from build123d import *

# Parameters (mm, degrees)
SKETCH_1_R          = 2
SKETCH_1_W          = 26
SKETCH_1_H          = 26
EXTRUDE_1_DEPTH     = 5
EXTRUDE_2_DEPTH     = 24
EXTRUDE_3_DEPTH     = 32
CUT_EXTRUDE_1_REACH = 71.979
SKETCH_3_R          = 6.35
CUT_EXTRUDE_2_REACH = 67.49
SKETCH_4_R          = 6.35
FILLET_2_R          = 3


with BuildPart() as part:
    # Sketch 1 → Extrude 1 (new body)
    with BuildSketch(Plane(origin=(0, 0, 0), x_dir=(1, 0, 0), z_dir=(0, 1, 0))):
        with BuildLine():
            Line((3, 0), (39, 0))
            ThreePointArc((39, 0), (41.121320344, 0.878679656), (42, 3))
            Line((42, 3), (42, 39))
            ThreePointArc((42, 39), (41.121320344, 41.121320344), (39, 42))
            Line((39, 42), (3, 42))
            ThreePointArc((3, 42), (0.878679656, 41.121320344), (0, 39))
            Line((0, 39), (0, 3))
            ThreePointArc((0, 3), (0.878679656, 0.878679656), (3, 0))
        make_face()
        with Locations(Location((5, 37, 0), (0, 0, 270))):
            Circle(SKETCH_1_R, mode=Mode.SUBTRACT)
        with Locations(Location((39, 37, 0), (0, 0, 270))):
            Circle(SKETCH_1_R, mode=Mode.SUBTRACT)
        with Locations(Location((5, 3, 0), (0, 0, 270))):
            Circle(SKETCH_1_R, mode=Mode.SUBTRACT)
        with Locations((21, 21)):
            Rectangle(SKETCH_1_W, SKETCH_1_H, mode=Mode.SUBTRACT)
    extrude(amount=EXTRUDE_1_DEPTH)

    # Sketch 2 → Extrude 2 (add)
    with BuildSketch(Plane(origin=(0, 5, 0), x_dir=(1, 0, 0), z_dir=(0, 1, 0))):
        Polygon((35.65, 34), (35.65, 42), (11.65, 42), (11.65, 34), (34, 34), align=None)
    extrude(amount=EXTRUDE_2_DEPTH)

    # Sketch 2_3 → Extrude 3 (add)
    with BuildSketch(Plane(origin=(0, 5, 0), x_dir=(1, 0, 0), z_dir=(0, 1, 0))):
        Polygon((8, 30.35), (0, 30.35), (0, 6.35), (8, 6.35), (8, 8), align=None)
    extrude(amount=EXTRUDE_3_DEPTH)

    # Sketch 3 → Cut-Extrude 1 (cut, up to next)
    with BuildSketch(Plane(origin=(0, 0, -42), x_dir=(-1, 0, 0), z_dir=(0, 0, -1)), mode=Mode.PRIVATE) as cut_extrude_1_sk1:
        with Locations((-25.65, 20)):
            Circle(SKETCH_3_R)
    cut_extrude_1_tool1 = extrude(cut_extrude_1_sk1.sketch, amount=-CUT_EXTRUDE_1_REACH, mode=Mode.PRIVATE) & part.part
    # Sketch 3 → Cut-Extrude 1 (cut, up to next)
    with BuildSketch(Plane(origin=(0, 0, -42), x_dir=(-1, 0, 0), z_dir=(0, 0, -1)), mode=Mode.PRIVATE) as cut_extrude_1_sk2:
        with BuildLine():
            Line((-30.008898944, 29), (-35.65, 29))
            Line((-35.65, 29), (-35.65, 20))
            ThreePointArc((-35.65, 20), (-34.123163206, 25.310885546), (-30.008898944, 29))
        make_face()
    cut_extrude_1_tool2 = extrude(cut_extrude_1_sk2.sketch, amount=-CUT_EXTRUDE_1_REACH, mode=Mode.PRIVATE) & part.part
    add(cut_extrude_1_tool1.solids().sort_by_distance((25.65, 20, -42))[0], mode=Mode.SUBTRACT)
    add(cut_extrude_1_tool2.solids().sort_by_distance((34.089564, 26.895646, -42))[0], mode=Mode.SUBTRACT)

    # Sketch 4 → Cut-Extrude 2 (cut, up to next)
    with BuildSketch(Plane(origin=(8, 0, 0), x_dir=(0, 0, -1), z_dir=(1, 0, 0)), mode=Mode.PRIVATE) as cut_extrude_2_sk1:
        with Locations((16.35, 28)):
            Circle(SKETCH_4_R)
    cut_extrude_2_tool1 = extrude(cut_extrude_2_sk1.sketch, amount=-CUT_EXTRUDE_2_REACH, mode=Mode.PRIVATE) & part.part
    # Sketch 4 → Cut-Extrude 2 (cut, up to next)
    with BuildSketch(Plane(origin=(8, 0, 0), x_dir=(0, 0, -1), z_dir=(1, 0, 0)), mode=Mode.PRIVATE) as cut_extrude_2_sk2:
        with BuildLine():
            Line((11.991101056, 37), (6.35, 37))
            Line((6.35, 37), (6.35, 28))
            ThreePointArc((6.35, 28), (7.876836794, 33.310885546), (11.991101056, 37))
        make_face()
    cut_extrude_2_tool2 = extrude(cut_extrude_2_sk2.sketch, amount=-CUT_EXTRUDE_2_REACH, mode=Mode.PRIVATE) & part.part
    add(cut_extrude_2_tool1.solids().sort_by_distance((8, 28, -16.35))[0], mode=Mode.SUBTRACT)
    add(cut_extrude_2_tool2.solids().sort_by_distance((8, 34.895646, -7.910436))[0], mode=Mode.SUBTRACT)

    # Fillet 2
    fillet_2_edges = [part.edges().sort_by_distance(p)[0] for p in [
        (4, 37, -11.991101056),
        (11.65, 17, -42),
        (11.65, 17, -34),
        (8, 21, -30.35),
        (0, 21, -30.35),
        (30.008898944, 29, -38),
    ]]
    fillet(fillet_2_edges, radius=FILLET_2_R)


solid = part.part
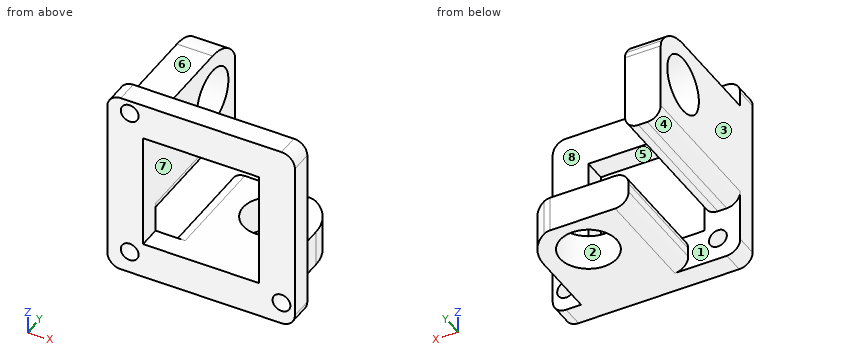
Build history of the part. All positions in model axes, mm. Face numbers are marked on the shaded views. A direction names the side the tool comes from. Coordinates: 2 decimals unless noted, no trailing zeros. Order: outer loops, then holes, each group sorted by start corner. A loop starts at its lowest first (then second) coordinate and runs counter-clockwise, first axis right, second up. Notation, with made-up numbers: (52, -9) -> (67, -9) arc R26 cw to (67, 21) -> close; hole circle Ø1 at (-27.5, 64.5). An arc over 180 degrees is marked (long way). One line per item, written item: value.
(1) Drop flat-ended pins along their axis: pin 1 Ø2 at (y, z) = (21.5, -38) entering from -X; pin 2 Ø4 at (y, z) = (21, -32) entering from -X; pin 3 Ø8.5 at (y, z) = (17.5, -27) entering from +X; pin 4 Ø8 at (x, z) = (9.5, -13) entering from +Y. Give the stop position or say it passes through.
Checked values:
pin 1: x = 11.65
pin 2: x = 1.59
pin 3: x = 8
pin 4: y = 37
(2) Mould opens along Y. For the marked faces 1, 2 and 3 say: pulls with the +Y half, pulls with the -Y half, needs draft (parallel to the pull), parting line crosses it, or undercut.
Checked values:
face 1: pulls with the +Y half
face 2: undercut
face 3: needs draft
(3) Slice it at C-C, the plane z = -16.35. List the corners of the cut face in (x, y), plus the area to 3 significant figures.
Checked values:
outline: (0, 0) -> (8, 0) -> (8, 21.65) -> (0, 21.65) -> close; (0, 34.35) -> (8, 34.35) -> (8, 37) -> (0, 37) -> close; (34, 0) -> (42, 0) -> (42, 5) -> (34, 5) -> close
area: 234 mm2
(4) Probe line 1 (X direction, y = 2, z = -37); line 2 (Z direction, x = 29.5, y = 3); line 3 (Y direction, x = 3.25, z = -16.35). List the from-to ranges inside material, lowest first. Write a range as [from, to].
Checked values:
line 1: [0, 3], [7, 37], [41, 42]
line 2: [-42, -34], [-8, 0]
line 3: [0, 21.65], [34.35, 37]
(5) Slice it at A-A, the plane y = 10.5. List the corners of the cut face in (x, z).
Checked values:
outline: (0, -27.35) arc R3 ccw to (3, -30.35) -> (5, -30.35) arc R3 ccw to (8, -27.35) -> (8, -6.35) -> (0, -6.35) -> close; (11.65, -39) arc R3 ccw to (14.65, -42) -> (35.65, -42) -> (35.65, -34) -> (14.65, -34) arc R3 ccw to (11.65, -37) -> close
(6) Slice it at D-D, the plane x = 25.65. List the corners of the cut face in (y, z).
Checked values:
outline: (0, -42) -> (13.65, -42) -> (13.65, -34) -> (0, -34) -> close; (0, -8) -> (5, -8) -> (5, 0) -> (0, 0) -> close; (26.35, -42) -> (29, -42) -> (29, -34) -> (26.35, -34) -> close
(7) Slice it at B-B, the plane x = 11. List the corners of the cut face in (y, z).
Checked values:
outline: (0, -42) -> (5, -42) -> (5, -34) -> (0, -34) -> close; (0, -8) -> (5, -8) -> (5, 0) -> (0, 0) -> close
(8) Tool access for the marked faces 4, 5, 6, 7 and 8: list every direction of +Z, -Z, +X, -X, +Y, -Y with a clear straight run to the whole face (end or side of a thin tool).
Checked values:
face 4: -Z, -X, +Y
face 5: +Y, -Y
face 6: +Z, +X, -X, +Y
face 7: +Y
face 8: +Z, +X, +Y
